Work out the finished part from the listing and answer in its coordinate system (mm). A direction names the side the tool comes from. Round coordinates to 2 decimals unless told otherwise and drop trailing zeros. Write each loop counter-clockwise with the first axis right and the second up, starting at its lowest first coordinate (ties: lowest second). Pieces come first, ordered by that corner, then holes. Notation, with made-up numbers: M 33,35 L 56,35 A21 cw 56,44 Z; hole C 83.5,35 d9. An arc over 180 degrees is marked long. Answer in a Markdown table with one row per item.
```python
from build123d import *

# Parameters (mm, degrees)
SKETCH008_W     = 62.5
SKETCH008_H     = 32.7
PAD007_DEPTH    = 2
SKETCH009_W     = 55.5
SKETCH009_H     = 28.7
PAD008_DEPTH    = 20.75
SKETCH010_R     = 7.25
POCKET001_DEPTH = 3
SKETCH011_R     = 1.5
POCKET002_DEPTH = 2
SKETCH012_W     = 23.9
SKETCH012_H     = 16
POCKET003_DEPTH = 2
SKETCH017_W     = 8.1
SKETCH017_H     = 4.75
POCKET004_DEPTH = 40
SKETCH018_W     = 10
SKETCH018_H     = 25
POCKET005_DEPTH = 2


with BuildPart() as part:
    # Sketch008 → Pad007 (new body)
    with BuildSketch(Plane.XY):
        Rectangle(SKETCH008_W, SKETCH008_H)
    extrude(amount=PAD007_DEPTH)

    # Sketch009 (on Face6 of Pad007) → Pad008 (join)
    with BuildSketch(Plane.XY.offset(2)):
        Polygon((-31.25, 16.35), (-26.25, 16.35), (31.25, 16.35), (31.25, 14.35), (31.25, -14.35), (31.25, -16.35), (-26.25, -16.35), (-31.25, -16.35), align=None)
        with Locations((1.5, 0)):
            Rectangle(SKETCH009_W, SKETCH009_H, mode=Mode.SUBTRACT)
    extrude(amount=PAD008_DEPTH)

    # Sketch010 (on Face15 of Pad008) → Pocket001 (cut)
    with BuildSketch(Plane.YZ.offset(-26.25)):
        with Locations((0, 12.375)):
            Circle(SKETCH010_R)
    extrude(amount=-POCKET001_DEPTH, mode=Mode.SUBTRACT)

    # Sketch011 (on Face21 of Pocket001) → Pocket002 (cut)
    with BuildSketch(Plane.YZ.offset(-29.25)):
        with Locations((0, 12.375)):
            Circle(SKETCH011_R)
    extrude(amount=-POCKET002_DEPTH, mode=Mode.SUBTRACT)

    # Sketch012 (on Face10 of Pocket002) → Pocket003 (cut)
    with BuildSketch(Plane.YZ.offset(31.25)):
        with Locations((0, 14.75)):
            Rectangle(SKETCH012_W, SKETCH012_H)
    extrude(amount=-POCKET003_DEPTH, mode=Mode.SUBTRACT)

    # Sketch017 → Pocket004 (cut)
    with BuildSketch(Plane.YZ):
        with Locations((0, 4.375)):
            Rectangle(SKETCH017_W, SKETCH017_H)
    extrude(amount=POCKET004_DEPTH, mode=Mode.SUBTRACT)

    # Sketch018 (on Face19 of Pad008) → Pocket005 (cut)
    with BuildSketch(Plane.XY.offset(2)):
        with Locations((-21.25, 0)):
            Rectangle(SKETCH018_W, SKETCH018_H)
        with Locations((-6.25, 0)):
            Rectangle(SKETCH018_W, SKETCH018_H)
    extrude(amount=-POCKET005_DEPTH, mode=Mode.SUBTRACT)


solid = part.part
```
1. The part is cut by section D-D (x = 2.5). Determine the outline of the cut face in (y, z).
Calculated:
| item | result |
|---|---|
| outline | M -16.35,0 L 16.35,0 L 16.35,22.75 L 14.35,22.75 L 14.35,2 L -14.35,2 L -14.35,22.75 L -16.35,22.75 Z |
2. Determine the mould class of faces 1 (the flat face through (-4.5, -14.5, 22.75)), 2 (the flat face through (0, 16.35, 11)), 3 (the flat face through (-16.25, 0, 1)) for opening direction Y: released by +Y, released by -Y, zero draft, split by the parting line, or undercut.
Calculated:
| item | result |
|---|---|
| face 1 | zero draft |
| face 2 | released by +Y |
| face 3 | undercut |
3. The part is cut by section A-A (y = -8). Determine the outline of the cut face in (x, z), plus the area to 3 significant figures.
Calculated:
| item | result |
|---|---|
| outline | M -31.25,0 L -26.25,0 L -26.25,22.75 L -31.25,22.75 Z; M -16.25,0 L -11.25,0 L -11.25,2 L -16.25,2 Z; M -1.25,0 L 31.25,0 L 31.25,6.75 L 29.25,6.75 L 29.25,2 L -1.25,2 Z |
| area | 198 mm² |
4. The part is cut by section B-B (y = 0). Determine the outline of the cut face in (x, z) (3 decimals), plus the area to 3 significant figures.
Calculated:
| item | result |
|---|---|
| outline | M -31.25,0 L -26.25,0 L -26.25,5.125 L -29.25,5.125 L -29.25,10.875 L -31.25,10.875 Z; M -31.25,13.875 L -29.25,13.875 L -29.25,19.625 L -26.25,19.625 L -26.25,22.75 L -31.25,22.75 Z; M -16.25,0 L -11.25,0 L -11.25,2 L -16.25,2 Z; M -1.25,0 L 31.25,0 L 31.25,2 L -1.25,2 Z |
| area | 139 mm² |
5. Consider line 1 along Z through (x, y) = (-30.25, 0) (3 decimals); line 2 along Y through (x, z) = (-6, 8); line 3 along X through (y, z) = (13, 18.5). Determine where each line is inside the solid, lowest interval first. Write a range as from..to.
Calculated:
| item | result |
|---|---|
| line 1 | z = 0..10.875, 13.875..22.75 |
| line 2 | y = -16.35..-14.35, 14.35..16.35 |
| line 3 | x = -31.25..-26.25, 29.25..31.25 |
6. A tool of negligible diameter and unlimited length cuts with its end or side. For faces 4 (the flat face through (-21, -12.5, 1)), 5 (the cylindrical face through (-30.24, -0.33, 10.91)), 6 (the flat face through (31.25, 0, 1)), 7 (the flat face through (30, 4.05, 4)), 8 (the flat face through (29.25, 13, 8)), from which of +Z, -Z, +X, -X, +Y, -Y can it reach the whole face along a straight path? Write none if from no direction.
Calculated:
| item | result |
|---|---|
| face 4 | +Z, -Z |
| face 5 | +X, -X |
| face 6 | +Z, -Z, +X, +Y, -Y |
| face 7 | +Z, +X |
| face 8 | +Z |
7. Given pin 1 (1.5 mm diameter, centred on x = -19, y = 13, fed in from +Z); pin 2 (11.5 mm diameter, centred on y = -3, z = 11.5, fed in from +X); pin 3 (0.6 mm diameter, centred on x = 30, y = -7, fed in from +Z); pin 4 (2 mm diameter, centred on y = -2, z = 19.5, fed in from +X), each flat-ended and moving along its own axis, determine where each tip first touches the part or whether it passes through.
Calculated:
| item | result |
|---|---|
| pin 1 | stops at z = 2 |
| pin 2 | stops at x = 31.25 |
| pin 3 | stops at z = 6.75 |
| pin 4 | stops at x = -26.25 |
8. The part is cut by section C-C (x = -20.5). Determine the outline of the cut face in (y, z), plus the area to 3 significant figures.
Calculated:
| item | result |
|---|---|
| outline | M -16.35,0 L -12.5,0 L -12.5,2 L -14.35,2 L -14.35,22.75 L -16.35,22.75 Z; M 12.5,0 L 16.35,0 L 16.35,22.75 L 14.35,22.75 L 14.35,2 L 12.5,2 Z |
| area | 98.4 mm² |
